from build123d import *

# Parameters (mm, degrees)
SKETCH1_W           = 184
SKETCH1_H           = 86
PLATE_DEPTH         = 10
BOSS_EXTRUDE1_DEPTH = 20
BOSS_EXTRUDE2_START = 15
BOSS_EXTRUDE2_DEPTH = 5
BOSS_EXTRUDE3_START = -15
BOSS_EXTRUDE3_DEPTH = 5
SKETCH3_R           = 8
CUT_EXTRUDE1_DEPTH  = 40
FILLET1_R           = 5


with BuildPart() as part:
    # Sketch1 → plate (new body)
    with BuildSketch(Plane(origin=(0, 0, 0), x_dir=(1, 0, 0), z_dir=(0, 1, 0))):
        Rectangle(SKETCH1_W, SKETCH1_H)
    extrude(amount=PLATE_DEPTH)

    # Sketch2 → Boss-Extrude1 (add, symmetric)
    with BuildSketch(Plane.XY):
        Polygon((-14, 10), (-14, 46), (-20, 46), (-20, 16), (-50, 16), (-50, 10), align=None)
        Polygon((50, 16), (50, 10), (14, 10), (14, 46), (20, 46), (20, 16), align=None)
    extrude(amount=BOSS_EXTRUDE1_DEPTH, both=True)

    # Sketch2<3> → Boss-Extrude2 (add)
    with BuildSketch(Plane.XY.offset(BOSS_EXTRUDE2_START)):
        Polygon((-20, 16), (-20, 31), (-35, 16), align=None)
        Polygon((35, 16), (20, 31), (20, 16), align=None)
    extrude(amount=BOSS_EXTRUDE2_DEPTH)

    # Sketch2<4> → Boss-Extrude3 (add)
    with BuildSketch(Plane.XY.offset(BOSS_EXTRUDE3_START)):
        Polygon((-20, 16), (-20, 31), (-35, 16), align=None)
        Polygon((35, 16), (20, 31), (20, 16), align=None)
    extrude(amount=-BOSS_EXTRUDE3_DEPTH)

    # Sketch3 → Cut-Extrude1 (cut)
    with BuildSketch(Plane.ZY.offset(20)):
        with Locations((0, 34)):
            Circle(SKETCH3_R)
    extrude(amount=-CUT_EXTRUDE1_DEPTH, mode=Mode.SUBTRACT)

    # Fillet1
    fillet1_edges = [part.edges().sort_by_distance(p)[0] for p in [
        (-17, 46, -20),
        (-17, 46, 20),
        (17, 46, 20),
        (17, 46, -20),
    ]]
    fillet(fillet1_edges, radius=FILLET1_R)


solid = part.part
The listing builds one solid part. Answer for the finished solid, in the listing's coordinates (mm). A direction names the side the tool comes from. Give positions to 0.01 mm unless a question says otherwise; leave off trailing zeros. Loops run counter-clockwise (first coordinate to the right, second up) from the corner with the lowest first, then second, coordinate; pieces in that order, holes last.
Item 1: A tool of negligible diameter and unlimited length cuts with its end or side. For faces 4 (the flat face through (-50, 13, 0)), 5 (the flat face through (-24, 20, 15)), 6 (the flat face through (24, 20, 15)), from which of +Z, -Z, +X, -X, +Y, -Y can it reach the whole face along a straight path? Write none if from no direction.
Derived:
face 4: +Z, -Z, -X, +Y
face 5: -X, +Y
face 6: +X, +Y
Item 2: Determine the mould class of faces 1 (the flat face through (14, 24, 0)), 2 (the cylindrical face through (-17, 44, -19)), 3 (the flat face through (20, 25, 0)) for opening direction Z: +Z half, -Z half, draft (parallel to the pull), parting line (faces both ways), or undercut.
Derived:
face 1: draft
face 2: -Z half
face 3: undercut
Item 3: A cutting plane is placed at C-C (y = 13.5). Give the vertices of the cut face in (x, z).
Derived:
outline: (-50, -20) - (-14, -20) - (-14, 20) - (-50, 20) - close; (14, -20) - (50, -20) - (50, 20) - (14, 20) - close
Item 4: A cutting plane is placed at A-A (z = 0). Give the vertices of the cut face in (x, y), then the cut area to 3 significant figures.
Derived:
outline: (-92, 0) - (92, 0) - (92, 10) - (50, 10) - (50, 16) - (20, 16) - (20, 26) - (14, 26) - (14, 10) - (-14, 10) - (-14, 26) - (-20, 26) - (-20, 16) - (-50, 16) - (-50, 10) - (-92, 10) - close; (-20, 42) - (-14, 42) - (-14, 46) - (-20, 46) - close; (14, 42) - (20, 42) - (20, 46) - (14, 46) - close
area: 2,440 mm2
Item 5: Each of these flat-tipped pins is pushed along its axis until it touches: pin 1 Ø16.5 at (x, y) = (-25.5, 26.5) entering from -Z; pin 2 Ø18.5 at (y, z) = (34, 0) entering from -X; pin 3 Ø18 at (y, z) = (21.5, -2.5) entering from -X. Where does it stop, or does it pass through?
Derived:
pin 1: stops at z = -20
pin 2: stops at x = -20
pin 3: stops at x = -50
Item 6: A cutting plane is placed at D-D (x = 42). Give the vertices of the cut face in (y, z).
Derived:
outline: (0, -43) - (10, -43) - (10, -20) - (16, -20) - (16, 20) - (10, 20) - (10, 43) - (0, 43) - close
Item 7: Find the intervals of material crossed by line 1 along Y through (x, z) = (15.35, 0); line 2 along X through (y, z) = (13.5, 6); line 3 along X through (y, z) = (44, 10), in increasing order.
Derived:
line 1: y = 0 to 26, 42 to 46
line 2: x = -50 to -14, 14 to 50
line 3: x = -20 to -14, 14 to 20
Item 8: A cutting plane is placed at B-B (y = 34). Give the vertices of the cut face in (x, z).
Derived:
outline: (-20, -20) - (-14, -20) - (-14, -8) - (-20, -8) - close; (-20, 8) - (-14, 8) - (-14, 20) - (-20, 20) - close; (14, -20) - (20, -20) - (20, -8) - (14, -8) - close; (14, 8) - (20, 8) - (20, 20) - (14, 20) - close
